Part model, mm, in its own coordinate system. Face numbers are marked on the shaded views. A direction names the side the tool comes from. Round coordinates to 2 decimals unless told otherwise and drop trailing zeros. Put each result on its own line as item: value. Start each with the question number.
1) Drop flat-ended pins along their axis: pin 1 Ø1 at (x, y) = (6, 1) entering from -Z; pin 2 Ø3 at (x, z) = (0, 0) entering from +Y; pin 3 Ø1.5 at (x, y) = (-10, 1.5) entering from -Z. Give the stop position or say it passes through.
2) Which spindle directions (+Z, -Z, +X, -X, +Y, -Y) get a long thin tool onto all of the face, cutting with end or side? Do the marked faces 1 and 2. Say none if no direction does.
3) Probe line 1 along Z through (x, y) = (-11.75, 0.8); line 2 along X through (y, z) = (2.2, 0). List the from-to ranges inside material, lowest first.
```python
from build123d import *

# Parameters (mm, degrees)
SKETCH1_R           = 15
BOSS_EXTRUDE1_DEPTH = 5
SKETCH2_R           = 2
CUT_EXTRUDE1_DEPTH  = 6
CUT_EXTRUDE2_DEPTH  = 10
CIRPATTERN1_COUNT   = 36


with BuildPart() as part:
    # Sketch1 → Boss-Extrude1 (new body)
    with BuildSketch(Plane(origin=(0, 0, 0), x_dir=(1, 0, 0), z_dir=(0, 1, 0))):
        Circle(SKETCH1_R)
    extrude(amount=BOSS_EXTRUDE1_DEPTH)

    # Sketch2 → Cut-Extrude1 (cut, through all)
    with BuildSketch(Plane(origin=(0, 5, 0), x_dir=(1, 0, 0), z_dir=(0, 1, 0))):
        Circle(SKETCH2_R)
    extrude(amount=-CUT_EXTRUDE1_DEPTH, mode=Mode.SUBTRACT)

    # Sketch3 → Cut-Extrude2 (cut)
    with BuildSketch(Plane(origin=(0, 5, 0), x_dir=(1, 0, 0), z_dir=(0, 1, 0))):
        Polygon((0, 12.8), (0.2, 12.8), (1, 14.966629547), (1, 18.114701451), (-1, 18.114701451), (-1, 14.966629547), (-0.2, 12.8), align=None)
    cut_extrude2 = extrude(amount=-CUT_EXTRUDE2_DEPTH, mode=Mode.SUBTRACT)

    # CirPattern1: Cut-Extrude2 ×36 about axis
    cirpattern1_axis = Axis((0, 0, 0), (0, 1, 0))
    for i in range(1, CIRPATTERN1_COUNT):
        add(cut_extrude2.rotate(cirpattern1_axis, i * 360 / CIRPATTERN1_COUNT), mode=Mode.SUBTRACT)


solid = part.part
```
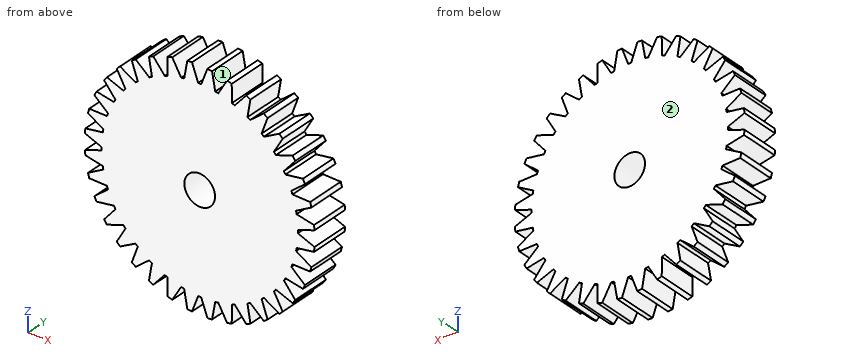
Recorded:
1. pin 1: stops at z = -13.72
1. pin 2: passes through
1. pin 3: stops at z = -10.82
2. face 1: +Z, +Y, -Y
2. face 2: +Z, -Z, +X, -X, +Y
3. line 1: z = -8.73 to -7.49, -6.32 to 6.32, 7.49 to 8.73
3. line 2: x = -12.8 to -2, 2 to 12.8
